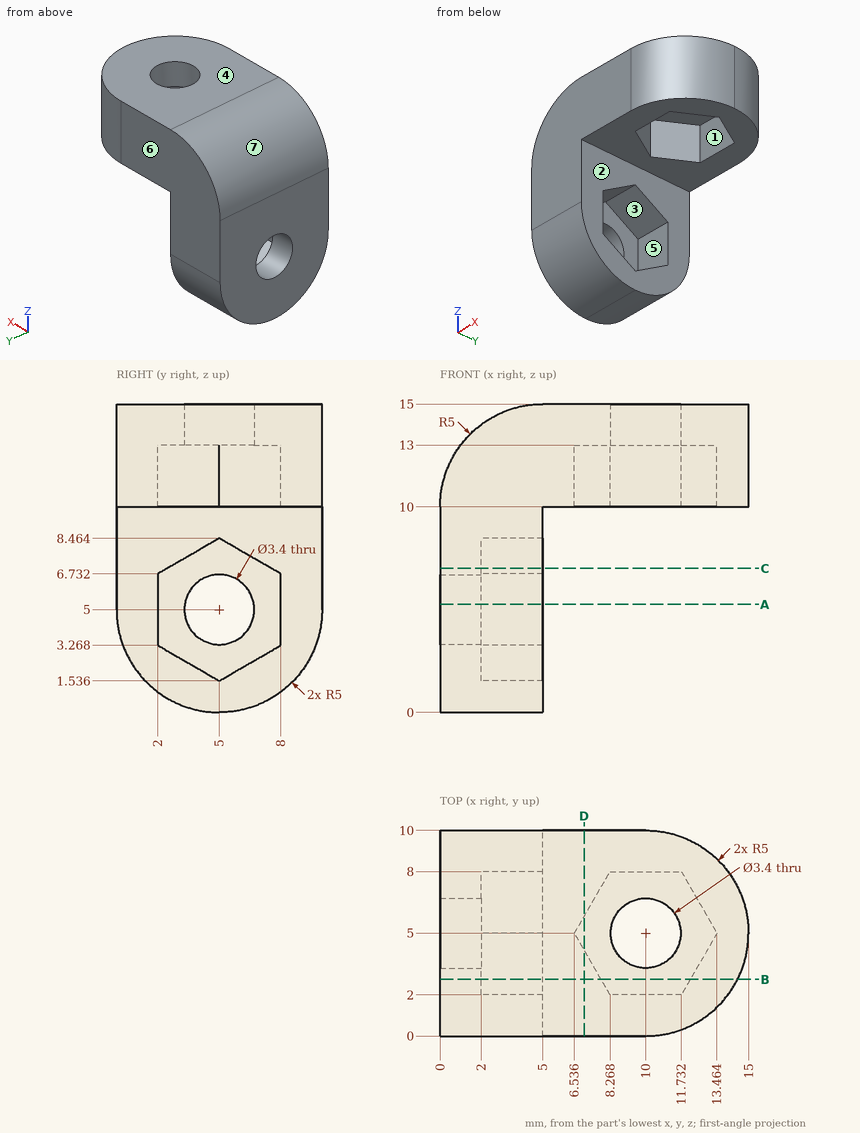
The figure shows three views and two pictorial views of one solid part (mm, origin at its lowest corner). Answer the questions. A direction names the side the tool comes from. Give positions to 0.01 mm unless a question says otherwise; leave off trailing zeros. Loops run counter-clockwise (first coordinate to the right, second up) from the corner with the lowest first, then second, coordinate; pieces in that order, holes last. Notation, with made-up numbers: (-35, -6.5) -> (-1, -6.5) arc R28 cw to (-1, 14.5) -> close; hole circle Ø3 at (33.25, 85.5). An arc over 180 degrees is marked (long way). Put each result on its own line as item: value. Start each with the question number.
Item 1: The part is cut by section D-D (x = 7). Give the vertices of the cut face in (y, z), then the cut area to 3 significant figures.
Item 2: Which of the six approach directions +Z, -Z, +X, -X, +Y, -Y give full straight-line access (tool end or side, diameter ignored) to the marked faces 1, 2, 3 and 4?
Item 3: The part is cut by section A-A (z = 5.25). Give the vertices of the cut face in (x, y).
Item 4: The part is cut by section B-B (y = 2.75). Give the vertices of the cut face in (x, z) (3 decimals), then the cut area to 3 significant figures.
Item 5: The mould has two halves that part along Z. Classify the marked faces 5, 6 and 7: released by +Z, released by -Z, zero draft, split by the parting line, or undercut.
Item 6: The part is cut by section C-C (z = 7). Give the vertices of the cut face in (x, y), then the cut area to 3 significant figures.
Item 7: Each of these flat-tipped pins is pushed along its axis until it touches: P1, Ø3, axis at x = 11.5, y = 3.5, coming from the -Z side; P2, Ø1, axis at x = 7, z = 7.5, coming from the -Y side; P3, Ø1.5, axis at x = 2.5, y = 7.5, coming from the +Z side; P4, Ø1, axis at y = 7, z = 11, coming from the -X side (3 decimals). Where does it stop, or does it pass through?
Item 8: Find the intervals of material crossed by L1, parallel to Y at x = 10, z = 14.25; L2, parallel to Z at x = 12.5, y = 1.75; L3, parallel to Z at x = 11.5, y = 7.5, in increasing order. Write a range as [from, to].
Answers below:
1. outline: (0, 10) -> (4.2, 10) -> (4.2, 13) -> (5.8, 13) -> (5.8, 10) -> (10, 10) -> (10, 15) -> (0, 15) -> close
1. area: 45.2 mm2
2. face 1: -Z
2. face 2: -Z, +X, +Y, -Y
2. face 3: +X
2. face 4: +Z, +X, -X, +Y, -Y
3. outline: (0, 0) -> (5, 0) -> (5, 2) -> (2, 2) -> (2, 3.32) -> (0, 3.32) -> close; (0, 6.68) -> (2, 6.68) -> (2, 8) -> (5, 8) -> (5, 10) -> (0, 10) -> close
4. outline: (0, 0.535) -> (5, 0.535) -> (5, 2.835) -> (2, 2.835) -> (2, 7.165) -> (5, 7.165) -> (5, 10) -> (7.835, 10) -> (7.835, 13) -> (12.165, 13) -> (12.165, 10) -> (14.465, 10) -> (14.465, 15) -> (5, 15) arc R5 ccw to (0, 10) -> close
4. area: 88.3 mm2
5. face 5: undercut
5. face 6: zero draft
5. face 7: released by +Z
6. outline: (0, 0) -> (5, 0) -> (5, 2.46) -> (2, 2.46) -> (2, 7.54) -> (5, 7.54) -> (5, 10) -> (0, 10) -> close
6. area: 34.8 mm2
7. P1: z = 10
7. P2: through
7. P3: z = 14.68
7. P4: x = 0.025
8. L1: [0, 3.3], [6.7, 10]
8. L2: [10, 15]
8. L3: [13, 15]
